Input: dimensioned drawing with shaded views. Units: mm. Origin: part minimum x, y, z. A direction names the side the tool comes from. Coordinates: 2 decimals unless noted, no trailing zeros. Order: outer loops, then holes, each group sorted by start corner. A loop starts at its lowest first (then second) coordinate and runs counter-clockwise, first axis right, second up.
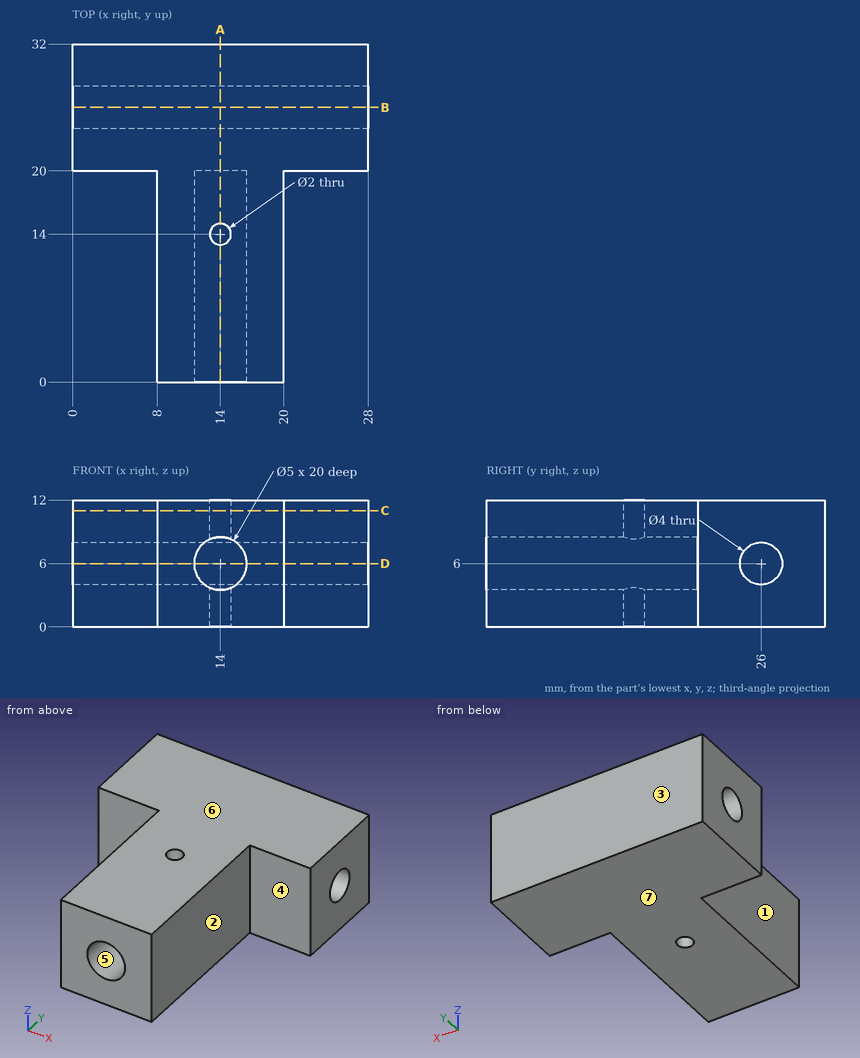
1. Access query for the marked faces 1, 2 and 3. Directions: +Z, -Z, +X, -X, +Y, -Y. A direction counts if a zero-diameter tool reaches every point of the face in a straight line with its end or side. Return the directions, or none.
Findings:
face 1: +Z, -Z, -X, -Y
face 2: +Z, -Z, +X, -Y
face 3: +Z, -Z, +X, -X, +Y
2. Section query D-D on z = 6. Return loops of the section in (x, y).
Findings:
outline: (0, 20) - (8, 20) - (8, 0) - (11.5, 0) - (11.5, 20) - (16.5, 20) - (16.5, 0) - (20, 0) - (20, 20) - (28, 20) - (28, 24) - (0, 24) - close; (0, 28) - (28, 28) - (28, 32) - (0, 32) - close
3. Pin query (flat end, axial travel): P1, Ø3, axis at y = 4.5, z = 7, coming from the +X side; P2, Ø2.5, axis at x = 2.5, z = 4.5, coming from the -Y side; P3, Ø1, axis at y = 5.5, z = 2.5, coming from the -X side. Return the tip coordinate at first contact, or that it passes through.
Findings:
P1: stops at x = 20
P2: stops at y = 20
P3: stops at x = 8
4. Section query B-B on y = 26. Return loops of the section in (x, z), plus the area to 3 significant figures.
Findings:
outline: (0, 0) - (28, 0) - (28, 4) - (0, 4) - close; (0, 8) - (28, 8) - (28, 12) - (0, 12) - close
area: 224 mm2
5. Ray query, line 1 (Y direction, x = 14, z = 10.8); line 2 (X direction, y = 15.5, z = 3.75); line 3 (X direction, y = 16.5, z = 5.25). Return the intervals inside material, ascending.
Findings:
line 1: y = 0 to 13, 15 to 32
line 2: x = 8 to 12.91, 15.09 to 20
line 3: x = 8 to 11.62, 16.38 to 20
6. Section query A-A on x = 14. Return loops of the section in (y, z).
Findings:
outline: (0, 0) - (13, 0) - (13, 3.5) - (0, 3.5) - close; (0, 8.5) - (13, 8.5) - (13, 12) - (0, 12) - close; (15, 0) - (32, 0) - (32, 12) - (15, 12) - (15, 8.5) - (20, 8.5) - (20, 3.5) - (15, 3.5) - close; hole circle Ø4 at (26, 6)
7. Draft query along Z for the marked faces 4, 5, 6 and 7. Return one class per face: released by +Z, released by -Z, zero draft, split by the parting line, or undercut.
Findings:
face 4: zero draft
face 5: undercut
face 6: released by +Z
face 7: released by -Z
8. Section query C-C on z = 11. Return loops of the section in (x, y).
Findings:
outline: (0, 20) - (8, 20) - (8, 0) - (20, 0) - (20, 20) - (28, 20) - (28, 32) - (0, 32) - close; hole circle Ø2 at (14, 14)
